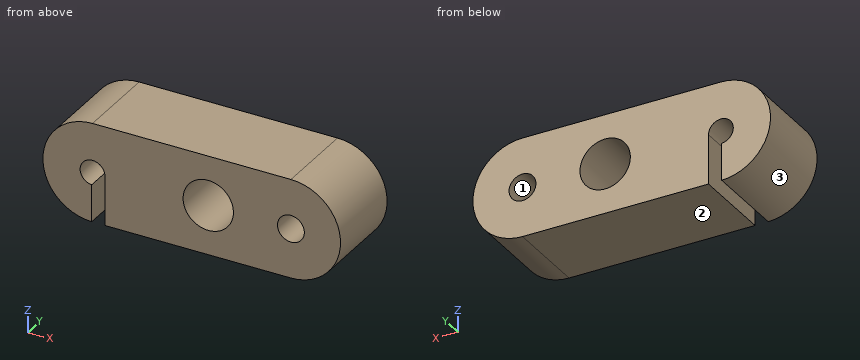
from build123d import *

# Parameters (mm, degrees)
SKETCH1_R           = 0.762
SKETCH1_R_2         = 0.4064
SKETCH1_R_3         = 0.375
BOSS_EXTRUDE1_DEPTH = 2.5
SKETCH2_W           = 0.4
SKETCH2_H           = 2.5
CUT_EXTRUDE1_DEPTH  = 6.361902647


with BuildPart() as part:
    # Sketch1 → Boss-Extrude1 (new body)
    with BuildSketch(Plane(origin=(0, 0, 0), x_dir=(1, 0, 0), z_dir=(0, 1, 0))):
        with BuildLine():
            Line((-3, 1.5), (3, 1.5))
            ThreePointArc((3, 1.5), (4.5, 0), (3, -1.5))
            Line((3, -1.5), (-3, -1.5))
            ThreePointArc((-3, -1.5), (-4.5, 0), (-3, 1.5))
        make_face()
        with Locations(Location((0.5, 0, 0), (0, 0, 270))):
            Circle(SKETCH1_R, mode=Mode.SUBTRACT)
        with Locations(Location((3, 0, 0), (0, 0, 270))):
            Circle(SKETCH1_R_2, mode=Mode.SUBTRACT)
        with Locations(Location((-3, 0, 0), (0, 0, 270))):
            Circle(SKETCH1_R_3, mode=Mode.SUBTRACT)
    extrude(amount=BOSS_EXTRUDE1_DEPTH)

    # Sketch2 → Cut-Extrude1 (cut, through all)
    with BuildSketch(Plane.XZ):
        with Locations((-2.825, -1.25)):
            Rectangle(SKETCH2_W, SKETCH2_H)
    extrude(amount=-CUT_EXTRUDE1_DEPTH, mode=Mode.SUBTRACT)


solid = part.part
Design review of the part built by this model. Coordinates are the model's own, in mm. Face numbers are marked on the shaded views. Round coordinates to 2 decimals unless told otherwise and drop trailing zeros. Loops run counter-clockwise (first coordinate to the right, second up) from the corner with the lowest first, then second, coordinate; pieces in that order, holes last. Notation, with made-up numbers: (-11.5, 80.25) - (23.5, 80.25) arc R23 ccw to (23.5, 94.25) - close; hole circle Ø11 at (-38, -38). An arc over 180 degrees is marked (long way). One line per question, with ' | ' between items.
1. For L1, parallel to X at y = 0.7, z = 0 (3 decimals); L2, parallel to X at y = 2.15, z = -0.65 (3 decimals); L3, parallel to X at y = 1.75, z = -0.5 (3 decimals), list the stretches that pass through material, from the lowest coordinate up. Write a range as [from, to].
Results are:
L1: x = [-4.5, -3.375], [-2.625, -0.262], [1.262, 2.594], [3.406, 4.5] | L2: x = [-4.352, -3.025], [-2.625, 0.102], [0.898, 4.352] | L3: x = [-4.414, -3.025], [-2.625, -0.075], [1.075, 4.414]
2. We need section B-B, the plane z = -0.55. State the section outline as (x, y) points (3 decimals), and give its area (3 significant figures).
Results are:
outline: (-4.396, 0) - (-3.025, 0) - (-3.025, 2.5) - (-4.396, 2.5) - close; (-2.625, 0) - (-0.027, 0) - (-0.027, 2.5) - (-2.625, 2.5) - close; (1.027, 0) - (4.396, 0) - (4.396, 2.5) - (1.027, 2.5) - close | area: 18.3 mm²
3. Draft analysis for pull direction X (two halves, no side actions). For the marked faces 1, 2 and 3, state which applies: released by +X, released by -X, zero draft, split by the parting line, or undercut.
Results are:
face 1: undercut | face 2: zero draft | face 3: released by -X
4. We need section A-A, the plane y = 1.3. State the section outline as (x, z) points (3 decimals).
Results are:
outline: (-3.025, -1.5) - (-3.025, -0.374) arc R0.375 cw (long way) to (-2.625, 0) - (-2.625, -1.5) - (3, -1.5) arc R1.5 ccw to (3, 1.5) - (-3, 1.5) arc R1.5 ccw to start; hole circle Ø1.524 at (0.5, 0); hole circle Ø0.813 at (3, 0)
5. Clearance check with flat-ended pins moving along their axes: P1, Ø0.9, axis at x = 0.5, z = 0, coming from the -Y side; P2, Ø0.9, axis at y = 1, z = -1, coming from the +X side. State where each tip first meets the part, or that it passes through.
Results are:
P1: passes through | P2: stops at x = 4.4
6. We need section D-D, the plane z = 0.5. State the section outline as (x, y) points.
Results are:
outline: (-4.41, 0) - (-0.08, 0) - (-0.08, 2.5) - (-4.41, 2.5) - close; (1.08, 0) - (4.41, 0) - (4.41, 2.5) - (1.08, 2.5) - close
7. We need section C-C, the plane x = 0.5. State the section outline as (y, z) points, and give its area (3 significant figures).
Results are:
outline: (0, -1.5) - (2.5, -1.5) - (2.5, -0.76) - (0, -0.76) - close; (0, 0.76) - (2.5, 0.76) - (2.5, 1.5) - (0, 1.5) - close | area: 3.69 mm²
